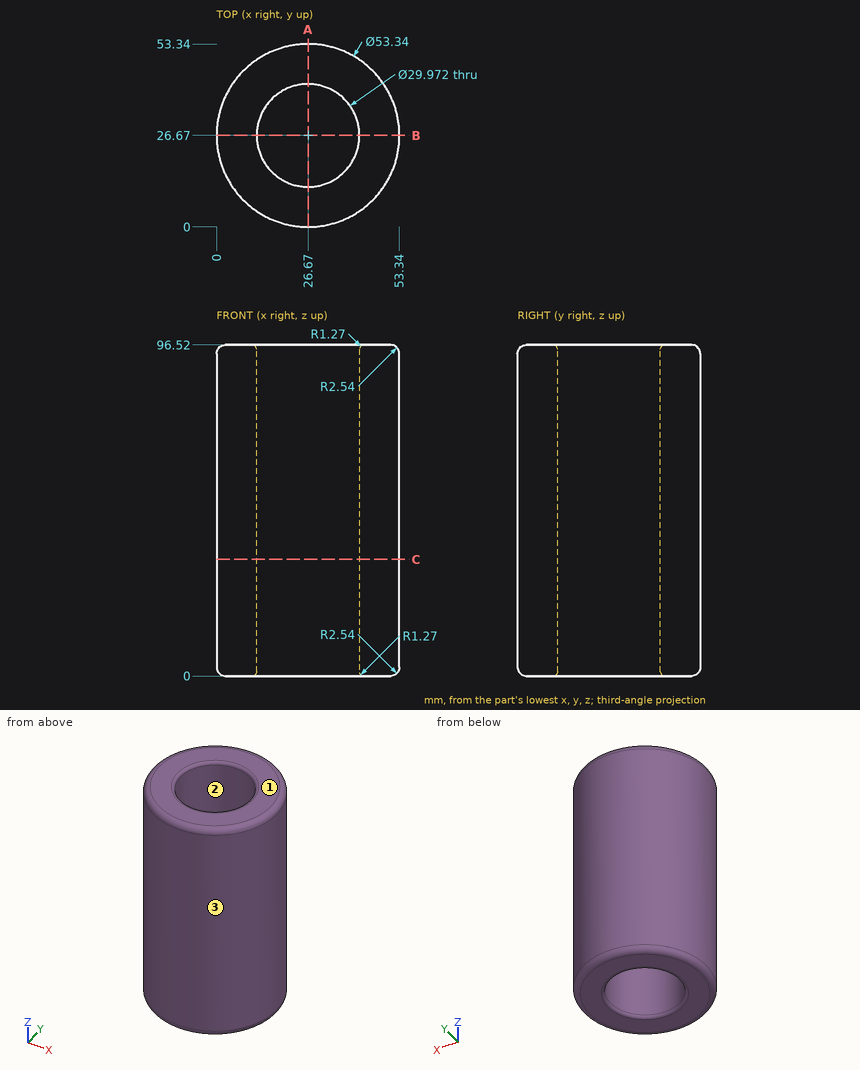
Answer from the drawing. Dimensions are ordinates in mm from the lowest x, y and z of the part. Coordinates: 2 decimals unless noted, no trailing zeros. Order: outer loops, then holes, each group sorted by start corner. A loop starts at its lowest first (then second) coordinate and runs counter-clockwise, first axis right, second up. Notation, with made-up numbers: (-19.75, 16) - (-4.75, 16) arc R19 ccw to (-4.75, 27) - close; hole circle Ø3 at (42.5, 15). An arc over 180 degrees is marked (long way). Answer as a JSON object with one key per item and string values. Group by question number.
Item 1: Flat-ended cylindrical pins translate along their axes: P1, Ø3, axis at x = 13.5, z = 85, coming from the -Y side; P2, Ø3, axis at x = 15, z = 30, coming from the +Y side; P3, Ø2, axis at y = 11.5, z = 49, coming from the -X side. Find the tip coordinate at first contact, or state that the pin passes through.
Item 2: Consider probe 1 along X at (y, z) = (26, 65); probe 2 along Y at (x, z) = (26.67, 50.5). Determine where each line is inside the solid, lowest interval first. Write a range as from..to.
Item 3: Section A-A (x = 26.67) is taken. Give the vertices of the cut face in (y, z).
Item 4: The mould has two halves that part along Y. Classify the marked faces 1, 2 and 3: +Y half, -Y half, draft (parallel to the pull), parting line (faces both ways), or undercut.
Item 5: Section C-C (z = 34) is taken. Give the vertices of the cut face in (x, y), plus the area to 3 significant figures.
Results are:
{
 "1": {"P1": "stops at y = 2.69", "P2": "stops at y = 51.32", "P3": "stops at x = 4.08"},
 "2": {"probe 1": "x = 0.01..11.7, 41.64..53.33", "probe 2": "y = 0..11.68, 41.66..53.34"},
 "3": {"outline": "(0, 2.54) arc R2.54 ccw to (2.54, 0) - (10.41, 0) arc R1.27 ccw to (11.68, 1.27) - (11.68, 95.25) arc R1.27 ccw to (10.41, 96.52) - (2.54, 96.52) arc R2.54 ccw to (0, 93.98) - close; (41.66, 1.27) arc R1.27 ccw to (42.93, 0) - (50.8, 0) arc R2.54 ccw to (53.34, 2.54) - (53.34, 93.98) arc R2.54 ccw to (50.8, 96.52) - (42.93, 96.52) arc R1.27 ccw to (41.66, 95.25) - close"},
 "4": {"face 1": "draft", "face 2": "undercut", "face 3": "parting line"},
 "5": {"outline": "circle Ø53.34 at (26.67, 26.67); hole circle Ø29.97 at (26.67, 26.67)", "area": "1,530 mm^2"}
}
